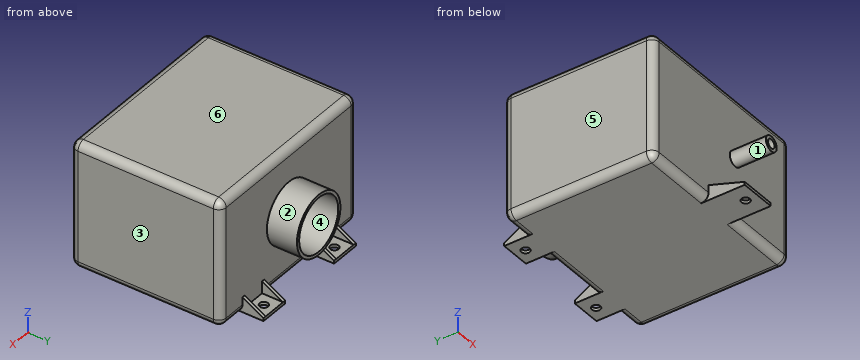
```python
from build123d import *

# Parameters (mm, degrees)
SKETCH1_W               = 158.75
SKETCH1_H               = 106.172
BOSS_EXTRUDE1_DEPTH     = 127
SKETCH2_R               = 25.4
BOSS_EXTRUDE2_DEPTH     = 25.4
SKETCH8_R               = 6.35
BOSS_EXTRUDE5_DEPTH     = 30.48
BOSS_EXTRUDE3_DEPTH     = 17.78
CUT_EXTRUDE2_DEPTH      = 196.580989608
CUT_EXTRUDE2_DEPTH_BACK = 196.580989608
BOSS_EXTRUDE4_DEPTH     = 30.48
SHELL1_START            = 2.54
SHELL1_OUTLINE_W        = 153.67
SHELL1_OUTLINE_H        = 101.092
SHELL1_DEPTH            = 121.92
SHELL1_START_2          = 124.46
SHELL1_2_OUTLINE_R      = 22.86
SHELL1_2_DEPTH          = 27.94
SHELL1_START_3          = -30.48
SHELL1_3_OUTLINE_R      = 3.81
SHELL1_3_DEPTH          = 33.02
CUT_EXTRUDE4_DEPTH      = 186.800131919
CUT_EXTRUDE4_DEPTH_BACK = 186.800131919
F_1_4_CLEARANCE_HOLE1_D = 7.14248
FILLET1_R               = 6.35


# Read off the part's stored shape, not the designer's step: Shell1
with BuildPart() as part:
    # Sketch1 → Boss-Extrude1 (new body)
    with BuildSketch(Plane(origin=(0, 0, 0), x_dir=(1, 0, 0), z_dir=(0, 1, 0))):
        Rectangle(SKETCH1_W, SKETCH1_H)
    extrude(amount=BOSS_EXTRUDE1_DEPTH)

    # Sketch2 → Boss-Extrude2 (add)
    with BuildSketch(Plane(origin=(0, 127, 0), x_dir=(1, 0, 0), z_dir=(0, 1, 0))):
        with Locations(Location((0, 0, 0), (0, 0, 270))):
            Circle(SKETCH2_R)
    extrude(amount=BOSS_EXTRUDE2_DEPTH)

    # Sketch8 → Boss-Extrude5 (add)
    with BuildSketch(Plane.XZ):
        with Locations(Location((15.875, 0, 0), (0, 0, 90))):
            Circle(SKETCH8_R)
    extrude(amount=BOSS_EXTRUDE5_DEPTH)

    # Sketch3 → Boss-Extrude3 (add)
    with BuildSketch(Plane(origin=(0, 127, 0), x_dir=(1, 0, 0), z_dir=(0, 1, 0))):
        Polygon((-53.975, 53.086), (-53.975, 40.386), (-51.435, 40.386), (-51.435, 50.546), (-31.115, 50.546), (-31.115, 40.386), (-28.575, 40.386), (-28.575, 53.086), align=None)
        Polygon((28.575, 53.086), (53.975, 53.086), (53.975, 40.386), (51.435, 40.386), (51.435, 50.546), (31.115, 50.546), (31.115, 40.386), (28.575, 40.386), align=None)
    extrude(amount=BOSS_EXTRUDE3_DEPTH)

    # Sketch5 → Cut-Extrude2 (cut, two sides: drawn at the far end of the back side and taken through both)
    with BuildSketch(Plane(origin=(31.115, 0, 0), x_dir=(0, 0, -1), z_dir=(1, 0, 0)).offset(-CUT_EXTRUDE2_DEPTH_BACK)):
        Polygon((40.386, 127), (50.546, 144.78), (40.386, 144.78), align=None)
    extrude(amount=CUT_EXTRUDE2_DEPTH + CUT_EXTRUDE2_DEPTH_BACK, mode=Mode.SUBTRACT)

    # Sketch7 → Boss-Extrude4 (add)
    with BuildSketch(Plane.XZ):
        Polygon((-15.24, -40.386), (-15.24, -53.086), (15.24, -53.086), (15.24, -40.386), (12.7, -40.386), (12.7, -50.546), (-12.7, -50.546), (-12.7, -40.386), align=None)
    extrude(amount=BOSS_EXTRUDE4_DEPTH)

    # Shell1 outline → Shell1 (cut)
    with BuildSketch(Plane(origin=(0, 0, 0), x_dir=(1, 0, 0), z_dir=(0, 1, 0)).offset(SHELL1_START)):
        Rectangle(SHELL1_OUTLINE_W, SHELL1_OUTLINE_H)
    extrude(amount=SHELL1_DEPTH, mode=Mode.SUBTRACT)

    # Shell1 2 outline → Shell1 2 (cut)
    with BuildSketch(Plane(origin=(0, 0, 0), x_dir=(1, 0, 0), z_dir=(0, 1, 0)).offset(SHELL1_START_2)):
        Circle(SHELL1_2_OUTLINE_R)
    extrude(amount=SHELL1_2_DEPTH, mode=Mode.SUBTRACT)

    # Shell1 3 outline → Shell1 3 (cut)
    with BuildSketch(Plane(origin=(0, 0, 0), x_dir=(1, 0, 0), z_dir=(0, 1, 0)).offset(SHELL1_START_3)):
        with Locations((15.875, 0)):
            Circle(SHELL1_3_OUTLINE_R)
    extrude(amount=SHELL1_3_DEPTH, mode=Mode.SUBTRACT)

    # Sketch9 → Cut-Extrude4 (cut, two sides: drawn at the far end of the back side and taken through both)
    with BuildSketch(Plane(origin=(-12.7, 0, 0), x_dir=(0, 0, -1), z_dir=(1, 0, 0)).offset(-CUT_EXTRUDE4_DEPTH_BACK)):
        Polygon((40.386, 0), (50.546, -30.48), (40.386, -30.48), align=None)
    extrude(amount=CUT_EXTRUDE4_DEPTH + CUT_EXTRUDE4_DEPTH_BACK, mode=Mode.SUBTRACT)

    # 1/4 Clearance Hole1 (through all)
    with Locations(Plane(origin=(-41.275, 135.89, -50.546), x_dir=(1, 0, 0), z_dir=(0, 0, 1))):
        with Locations((0, 0), (82.55, 0), (41.275, -156.21)):
            Hole(F_1_4_CLEARANCE_HOLE1_D / 2)

    # Fillet1
    fillet1_edges = [part.edges().sort_by_distance(p)[0] for p in [
        (-47.3075, 0, -53.086),
        (79.375, 127, 0),
        (66.675, 127, -53.086),
        (-66.675, 127, -53.086),
        (0, 127, -53.086),
        (-79.375, 127, 0),
        (47.3075, 0, -53.086),
        (79.375, 0, 0),
        (0, 0, 53.086),
        (-79.375, 0, 0),
        (-79.375, 63.5, -53.086),
        (79.375, 63.5, -53.086),
        (79.375, 63.5, 53.086),
        (-79.375, 63.5, 53.086),
        (0, 127, 53.086),
    ]]
    fillet(fillet1_edges, radius=FILLET1_R)


solid = part.part
```
The listing builds one solid part. Answer for the finished solid, in the listing's coordinates (mm). Face numbers are marked on the shaded views. A direction names the side the tool comes from. Round coordinates to 2 decimals unless told otherwise and drop trailing zeros. Order: outer loops, then holes, each group sorted by start corner. A loop starts at its lowest first (then second) coordinate and runs counter-clockwise, first axis right, second up. Notation, with made-up numbers: (64.5, -29.75) -> (99.5, -29.75) arc R17 cw to (99.5, -17.75) -> close; hole circle Ø8 at (13.25, -5.75). An arc over 180 degrees is marked (long way). Answer as CSV lines item,"result".
Q1. A cutting plane is placed at A-A on x = 0. Determine the outline of the cut face in (y, z), plus the area to 3 significant figures.
Computed values:
outline,"(-30.48, -53.09) -> (-23.89, -53.09) -> (-23.89, -50.55) -> (-30.48, -50.55) -> close; (-16.75, -53.09) -> (120.65, -53.09) arc R6.35 ccw to (127, -46.74) -> (127, -25.4) -> (152.4, -25.4) -> (152.4, -22.86) -> (124.46, -22.86) -> (124.46, -50.55) -> (2.54, -50.55) -> (2.54, 50.55) -> (124.46, 50.55) -> (124.46, 22.86) -> (152.4, 22.86) -> (152.4, 25.4) -> (127, 25.4) -> (127, 46.74) arc R6.35 ccw to (120.65, 53.09) -> (6.35, 53.09) arc R6.35 ccw to (0, 46.74) -> (0, -50.55) -> (-16.75, -50.55) -> close"
area,"1,200 mm^2"
Q2. A cutting plane is placed at D-D on x = -42.5. Determine the outline of the cut face in (y, z).
Computed values:
outline,"(0, -46.74) arc R6.35 ccw to (6.35, -53.09) -> (132.54, -53.09) -> (132.54, -50.55) -> (127, -50.55) -> (127, 46.74) arc R6.35 ccw to (120.65, 53.09) -> (6.35, 53.09) arc R6.35 ccw to (0, 46.74) -> close; (139.24, -53.09) -> (144.78, -53.09) -> (144.78, -50.55) -> (139.24, -50.55) -> close; hole (2.54, -50.55) -> (124.46, -50.55) -> (124.46, 50.55) -> (2.54, 50.55) -> close"
Q3. A cutting plane is placed at C-C on z = 0. Determine the outline of the cut face in (x, y) (3 decimals).
Computed values:
outline,"(-79.375, 6.35) arc R6.35 ccw to (-73.025, 0) -> (9.525, 0) -> (9.525, -30.48) -> (12.065, -30.48) -> (12.065, 2.54) -> (-76.835, 2.54) -> (-76.835, 124.46) -> (-22.86, 124.46) -> (-22.86, 152.4) -> (-25.4, 152.4) -> (-25.4, 127) -> (-73.025, 127) arc R6.35 ccw to (-79.375, 120.65) -> close; (19.685, -30.48) -> (22.225, -30.48) -> (22.225, 0) -> (73.025, 0) arc R6.35 ccw to (79.375, 6.35) -> (79.375, 120.65) arc R6.35 ccw to (73.025, 127) -> (25.4, 127) -> (25.4, 152.4) -> (22.86, 152.4) -> (22.86, 124.46) -> (76.835, 124.46) -> (76.835, 2.54) -> (19.685, 2.54) -> close"
Q4. For a pull along Z with two mould halves and no side action, classify the marked faces 4, 5 and 6 as +Z half, -Z half, draft (parallel to the pull), parting line (faces both ways), or undercut.
Computed values:
face 4,"undercut"
face 5,"draft"
face 6,"+Z half"
Q5. Consider line 1 (X direction, y = 135.89, z = -51.25) (3 decimals); line 2 (Z direction, x = -67.5, y = 50.5); line 3 (X direction, y = 138.5, z = 0). Determine where each line is inside the solid, lowest interval first. Write a range as from..to.
Computed values:
line 1,"x = -53.975..-44.846, -37.704..-28.575, 28.575..37.704, 44.846..53.975"
line 2,"z = -53.09..-50.55, 50.55..53.09"
line 3,"x = -25.4..-22.86, 22.86..25.4"
Q6. Given pin 1 (14 mm diameter, centred on y = 136, z = -45.5, fed in from +X) (3 decimals); pin 2 (9 mm diameter, centred on x = 46.5, y = 135.5, fed in from +Z); pin 3 (1 mm diameter, centred on x = -3, z = 16, fed in from -Y), each flat-ended and moving along its own axis, determine where each tip first touches the part or whether it passes through.
Computed values:
pin 1,"stops at x = 53.975"
pin 2,"stops at z = -50.55"
pin 3,"stops at y = 0"
Q7. A cutting plane is placed at B-B on y = 70.5. Determine the outline of the cut face in (x, z) (3 decimals), plus the area to 3 significant figures.
Computed values:
outline,"(-79.375, -46.736) arc R6.35 ccw to (-73.025, -53.086) -> (73.025, -53.086) arc R6.35 ccw to (79.375, -46.736) -> (79.375, 46.736) arc R6.35 ccw to (73.025, 53.086) -> (-73.025, 53.086) arc R6.35 ccw to (-79.375, 46.736) -> close; hole (-76.835, -50.546) -> (76.835, -50.546) -> (76.835, 50.546) -> (-76.835, 50.546) -> close"
area,"1,290 mm^2"
Q8. Which of the six approach directions +Z, -Z, +X, -X, +Y, -Y give full straight-line access (tool end or side, diameter ignored) to the marked faces 1, 2 and 3?
Computed values:
face 1,"-Y"
face 2,"+Y"
face 3,"+Z, -Z, +X, +Y, -Y"
